from build123d import *

# Parameters (mm, degrees)
BOSS_EXTRUDE1_DEPTH      = 5
BOSS_EXTRUDE1_DEPTH_BACK = 5
M5_CLEARANCE_HOLE1_D     = 5.3
M5_CLEARANCE_HOLE1_DEPTH = 23.08
M5_CLEARANCE_HOLE1_TIP   = 1.59228064


with BuildPart() as part:
    # Sketch1 → Boss-Extrude1 (new body, two sides)
    with BuildSketch(Plane.XY) as boss_extrude1_sk:
        Polygon((3, 2.5), (-3, 2.5), (-3, 1.5), (-5, 1.5), (-5, 0.5), (-2, -2.5), (2, -2.5), (5, 0.5), (5, 1.5), (3, 1.5), align=None)
    extrude(amount=BOSS_EXTRUDE1_DEPTH)
    extrude(boss_extrude1_sk.sketch, amount=-BOSS_EXTRUDE1_DEPTH_BACK)

    # M5 Clearance Hole1
    with Locations(Plane(origin=(0, 2.5, 0), x_dir=(1, 0, 0), z_dir=(0, 1, 0))):
        with Locations((0, 0)):
            Hole(M5_CLEARANCE_HOLE1_D / 2, depth=M5_CLEARANCE_HOLE1_DEPTH)
            with Locations((0, 0, -(M5_CLEARANCE_HOLE1_DEPTH + M5_CLEARANCE_HOLE1_TIP / 2))):  # 118° drill point
                Cone(0, M5_CLEARANCE_HOLE1_D / 2, M5_CLEARANCE_HOLE1_TIP, mode=Mode.SUBTRACT)


solid = part.part
The model under review builds one solid part; all positions refer to its coordinate system, in mm. A direction names the side the tool comes from. Round coordinates to 2 decimals unless told otherwise and drop trailing zeros. Loops run counter-clockwise (first coordinate to the right, second up) from the corner with the lowest first, then second, coordinate; pieces in that order, holes last. Notation, with made-up numbers: M -2.5,75.5 L 45.5,75.5 A20 ccw 45.5,83.5 Z; hole C 53,17 d8. An arc over 180 degrees is marked long. Answer as CSV lines item,"result". Start each with the question number.
Item 1: Consider section A-A (z = 0). Write out the cut boundary in (x, y).
Item 2: Consider section B-B (x = 1). Write out the cut boundary in (y, z), then the cut area to 3 significant figures.
Item 3: Consider section D-D (y = 1.65). Write out the cut boundary in (x, z).
Item 4: Insertion check: P1, Ø1, axis at x = -4, z = -0.5, coming from the +Y side; P2, Ø0.8, axis at y = 2, z = 1, coming from the +X side; P3, Ø0.5, axis at y = 2, z = 2.5, coming from the -X side; P4, Ø2, axis at y = 2, z = -0.5, coming from the +X side. Each pin has a flat end and moves straight along its axis. Give the tip position at first contact, or say it passes through.
Item 5: For faces 1 (the face through (-5, 1, 0)), 2 (the face through (3, 2, 0)), 3 (the face through (-4, 1.5, 0)), list the 3-axis set-ups (+Z, -Z, +X, -X, +Y, -Y) from which the entire face can be reached by the end or side of a thin tool; tool diameter is ignored.
Item 6: Mouldability with a two-part tool opening along Z and no side actions: class faces 4 (the face through (0, 0, 5)), 5 (the face through (2.647, -0.035, -0.117)), 6 (the face through (0, -2.5, -4)) as released by +Z, released by -Z, zero draft, split by the parting line, or undercut.
Item 7: Consider section C-C (z = 3). Write out the cut boundary in (x, y), then the cut area to 3 significant figures.
Item 8: Wall thickness on line 1 (Z direction, x = -2, y = 1.15); line 2 (Z direction, x = 0, y = 1.4); line 3 (Y direction, x = 2.5, z = 3.25): over which ranges is each line inside the solid? List them lowest first. Write a range as [from, to].
Answer:
1,outline,"M -5,0.5 L -2.65,-1.85 L -2.65,2.5 L -3,2.5 L -3,1.5 L -5,1.5 Z; M 2.65,-1.85 L 5,0.5 L 5,1.5 L 3,1.5 L 3,2.5 L 2.65,2.5 Z"
2,outline,"M -2.5,-5 L 2.5,-5 L 2.5,-2.45 L -2.5,-2.45 Z; M -2.5,2.45 L 2.5,2.45 L 2.5,5 L -2.5,5 Z"
2,area,"25.5 mm^2"
3,outline,"M -3,-5 L 3,-5 L 3,5 L -3,5 Z; hole C 0,0 d5.3"
4,P1,"stops at y = 1.5"
4,P2,"stops at x = 3"
4,P3,"stops at x = -3"
4,P4,"stops at x = 5"
5,face 1,"+Z, -Z, -X, +Y, -Y"
5,face 2,"+Z, -Z, +X, +Y"
5,face 3,"+Z, -Z, -X, +Y"
6,face 4,"released by +Z"
6,face 5,"undercut"
6,face 6,"zero draft"
7,outline,"M -5,0.5 L -2,-2.5 L 2,-2.5 L 5,0.5 L 5,1.5 L 3,1.5 L 3,2.5 L -3,2.5 L -3,1.5 L -5,1.5 Z"
7,area,"37.0 mm^2"
8,line 1,"z = [-5, -1.74], [1.74, 5]"
8,line 2,"z = [-5, -2.65], [2.65, 5]"
8,line 3,"y = [-2, 2.5]"
